Geometry check sheet. Reference: the model listing, model coordinates, mm. Face numbers are marked on the shaded views. A direction names the side the tool comes from. Give positions to 0.01 mm unless a question says otherwise; leave off trailing zeros. Order: outer loops, then holes, each group sorted by start corner. A loop starts at its lowest first (then second) coordinate and runs counter-clockwise, first axis right, second up. Notation, with made-up numbers: M 44.5,-35 L 103.5,-35 A21 cw 103.5,-14 Z; hole C -15.75,17.25 d10. An arc over 180 degrees is marked long. Answer as CSV lines item,"result".
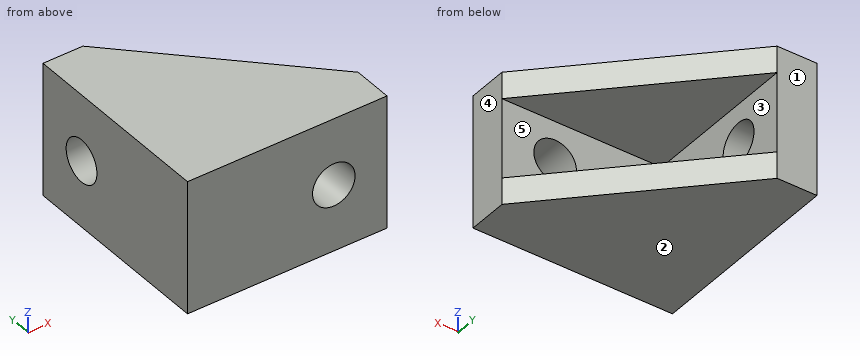
from build123d import *

# Parameters (mm, degrees)
BOSS_EXTRUDE1_DEPTH = 3
BOSS_EXTRUDE3_DEPTH = 2
SKETCH2_R           = 1.6
CUT_EXTRUDE1_DEPTH  = 4


with BuildPart() as part:
    # Sketch1 → Boss-Extrude1 (new body)
    with BuildSketch(Plane.XY):
        Polygon((0, 0), (0, 15), (3, 15), (3, 3), (15, 3), (15, 0), align=None)
    extrude(amount=BOSS_EXTRUDE1_DEPTH)

    # Sketch1_4 → Boss-Extrude3 (add)
    with BuildSketch(Plane.XY):
        Polygon((0, 15), (0, 0), (15, 0), (15, 3), (3, 3), (3, 15), align=None)
        Polygon((15, 3), (3, 15), (3, 3), align=None)
    extrude(amount=-BOSS_EXTRUDE3_DEPTH)

    # Mirror1: part across plane


with BuildPart() as part_1:
    add(part.part)
    add(part.part.mirror(Plane.XY.offset(3)))

    # Sketch2 → Cut-Extrude1 (cut, through all)
    with BuildSketch(Plane(origin=(3, 0, 0), x_dir=(0, 0, -1), z_dir=(1, 0, 0))):
        with Locations((-3, 11)):
            Circle(SKETCH2_R)
    cut_extrude1 = extrude(amount=-CUT_EXTRUDE1_DEPTH, mode=Mode.SUBTRACT)

    # Mirror2: Cut-Extrude1 across plane
    add(cut_extrude1.mirror(Plane(origin=(0, 0, 0), x_dir=(0, 0, 1), z_dir=(0.707106781, -0.707106781, 0))), mode=Mode.SUBTRACT)


solid = part_1.part
(1) Section check B-B on y = 11. Enter the section's corners in (x, z).
The answers:
outline,"M 0,-2 L 7,-2 L 7,0 L 3,0 L 3,1.4 L 0,1.4 Z; M 0,4.6 L 3,4.6 L 3,6 L 7,6 L 7,8 L 0,8 Z"
(2) Section check C-C on x = 4.5. Enter the section's corners in (y, z).
The answers:
outline,"M 0,-2 L 13.5,-2 L 13.5,0 L 3,0 L 3,6 L 13.5,6 L 13.5,8 L 0,8 Z"
(3) Tool access check on the marked faces 4 and 5. Record the directions out of +Z, -Z, +X, -X, +Y, -Y that give a thin tool (end or side, any length) a straight path to the whole face; none if there is none.
The answers:
face 4,"+Z, -Z, +X, +Y, -Y"
face 5,"+X, +Y"
(4) Section check A-A on z = 3. Enter the section's corners in (x, y).
The answers:
outline,"M 0,0 L 9.4,0 L 9.4,3 L 3,3 L 3,9.4 L 0,9.4 Z; M 0,12.6 L 3,12.6 L 3,15 L 0,15 Z; M 12.6,0 L 15,0 L 15,3 L 12.6,3 Z"
(5) Section check D-D on y = 7.25. Enter the section's corners in (x, z), then the cut area to 3 significant figures.
The answers:
outline,"M 0,-2 L 10.75,-2 L 10.75,0 L 3,0 L 3,6 L 10.75,6 L 10.75,8 L 0,8 Z"
area,"61.0 mm2"
(6) Gauge pin test, flat ends, axial feed: P1, Ø2, axis at y = 6, z = -0.5, coming from the +X side; P2, Ø2, axis at y = 10, z = 2, coming from the +X side; P3, Ø5, axis at y = 6.5, z = 6, coming from the +X side. Record the tip position at first contact, or that the pin passes through.
The answers:
P1,"stops at x = 13"
P2,"stops at x = 3"
P3,"stops at x = 14"
(7) Draft check along Z on the marked faces 1, 2 and 3. Enter one of: +Z half, -Z half, draft (parallel to the pull), parting line (faces both ways), or undercut.
The answers:
face 1,"draft"
face 2,"-Z half"
face 3,"undercut"
(8) Material ranges on line 1 (X direction, y = 1.15, z = 3); line 2 (Z direction, x = 10, y = 6.5), recorded low to high.
The answers:
line 1,"x = 0 to 9.4, 12.6 to 15"
line 2,"z = -2 to 0, 6 to 8"
